from build123d import *

# Parameters (mm, degrees)
SKETCH2_W           = 5
SKETCH2_H           = 3
BOSS_EXTRUDE2_DEPTH = 10
BOSS_EXTRUDE3_DEPTH = 5


with BuildPart() as part:
    # Sketch2 → Boss-Extrude2 (new body)
    with BuildSketch(Plane(origin=(0, 0, 0), x_dir=(1, 0, 0), z_dir=(0, 1, 0))):
        Polygon((0, 40.223426607), (0, 50.279283258), (-20.111713303, 34.834509269), (-25.139641629, 43.543136586), (-34.834509269, 20.111713303), (-43.543136586, 25.139641629), (-40.223426607, 0), (-50.279283258, 0), (-34.834509269, -20.111713303), (-43.543136586, -25.139641629), (-20.111713303, -34.834509269), (-25.139641629, -43.543136586), (0, -40.223426607), (0, -50.279283258), (20.111713303, -34.834509269), (25.139641629, -43.543136586), (34.834509269, -20.111713303), (43.543136586, -25.139641629), (40.223426607, 0), (50.279283258, 0), (34.834509269, 20.111713303), (43.543136586, 25.139641629), (20.111713303, 34.834509269), (25.139641629, 43.543136586), align=None)
        Rectangle(SKETCH2_W, SKETCH2_H, mode=Mode.SUBTRACT)
    extrude(amount=BOSS_EXTRUDE2_DEPTH)

    # Sketch3 → Boss-Extrude3 (add)
    with BuildSketch(Plane(origin=(0, 10, 0), x_dir=(1, 0, 0), z_dir=(0, 1, 0))):
        Polygon((0, 35.761861209), (-3.15, 6.933446407), (3.15, 6.933446407), align=None)
    extrude(amount=BOSS_EXTRUDE3_DEPTH)


solid = part.part
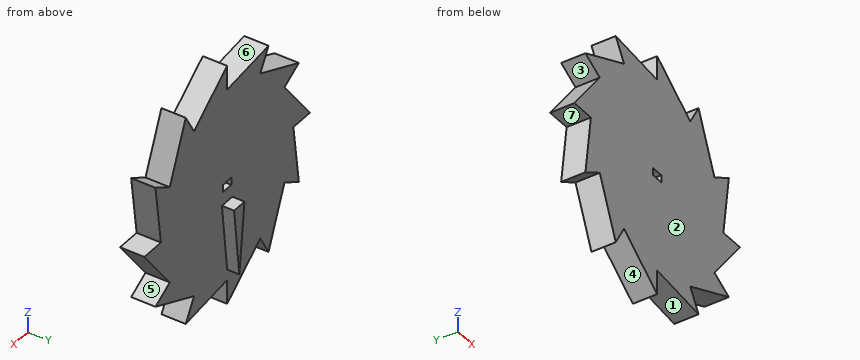
CAD build for the part. Positions are in the model's coordinates, mm. Face numbers are marked on the shaded views. A direction names the side the tool comes from. Give positions to 0.01 mm unless a question says otherwise; leave off trailing zeros. Write each loop counter-clockwise with the first axis right and the second up, starting at its lowest first coordinate (ties: lowest second). Pieces come first, ordered by that corner, then holes. Notation, with made-up numbers: (-30, -28.75) - (-12, -28.75) arc R36 ccw to (-12, 5.25) - close; hole circle Ø4 at (-11.75, 19.5). An arc over 180 degrees is marked (long way). Answer as CSV lines item,"result".
Q1. Band-saw the part on A-A (y = 7.5). Give the cut face in (x, z), and give its area (3 significant figures).
Result set:
outline,"(-50.28, 0) - (-40.22, 0) - (-43.54, -25.14) - (-34.83, -20.11) - (-25.14, -43.54) - (-20.11, -34.83) - (0, -50.28) - (0, -40.22) - (25.14, -43.54) - (20.11, -34.83) - (43.54, -25.14) - (34.83, -20.11) - (50.28, 0) - (40.22, 0) - (43.54, 25.14) - (34.83, 20.11) - (25.14, 43.54) - (20.11, 34.83) - (0, 50.28) - (0, 40.22) - (-25.14, 43.54) - (-20.11, 34.83) - (-43.54, 25.14) - (-34.83, 20.11) - close; hole (-2.5, -1.5) - (2.5, -1.5) - (2.5, 1.5) - (-2.5, 1.5) - close"
area,"6,050 mm²"
Q2. Drill centre lines: line 1 (Y direction, x = -21, z = 5); line 2 (Z direction, x = -35.5, y = 2.25); line 3 (Z direction, x = 35.5, y = 6.75). Where is each one in solid material? Low to high. Write a range as from..to.
Result set:
line 1,"0..10"
line 2,"-20.5..19.25, 20.5..28.47"
line 3,"-28.47..-20.5, -19.25..20.5"
Q3. Flat gauge pins, fed straight in: pin 1 Ø8 at (y, z) = (3.5, 42.5) entering from -X; pin 2 Ø5 at (y, z) = (5.5, -44.5) entering from +X; pin 3 Ø5.5 at (x, y) = (-0.5, 4.5) entering from -Z; pin 4 Ø6 at (x, y) = (31.5, 13.5) entering from -Z. Where does each tip first touch, or does it go through?
Result set:
pin 1,"x = -25.14"
pin 2,"x = 25.14"
pin 3,"z = -50.28"
pin 4,"through"
Q4. Pull direction Z, two halves, no side cores. Call the marked faces 1, 2 and 3: released by +Z, released by -Z, zero draft, split by the parting line, or undercut.
Result set:
face 1,"released by -Z"
face 2,"zero draft"
face 3,"undercut"
Q5. 3-axis set-ups, long thin cutter, end or side, ignore diameter. For the marked faces 4, 5, 6 and 7: which of +Z, -Z, +X, -X, +Y, -Y reach the whole face in a straight line?
Result set:
face 4,"-Z, +Y, -Y"
face 5,"+X, +Y, -Y"
face 6,"+Z, +Y, -Y"
face 7,"-X, +Y, -Y"
Q6. Band-saw the part on D-D (z = -11.5). Give the cut face in (x, y), and give its area (3 significant figures).
Result set:
outline,"(-41.74, 0) - (41.45, 0) - (41.45, 10) - (2.65, 10) - (2.65, 15) - (-2.65, 15) - (-2.65, 10) - (-41.74, 10) - close"
area,"858 mm²"
Q7. Band-saw the part on C-C (x = -23). Give the cut face in (y, z), and give its area (3 significant figures).
Result set:
outline,"(0, -39.84) - (10, -39.84) - (10, 33.64) - (0, 33.64) - close; (0, 39.84) - (10, 39.84) - (10, 43.26) - (0, 43.26) - close"
area,"769 mm²"
Q8. Band-saw the part on B-B (z = -37.5). Give the cut face in (x, y), and give its area (3 significant figures).
Result set:
outline,"(-27.64, 0) - (-21.65, 0) - (-21.65, 10) - (-27.64, 10) - close; (-16.64, 0) - (21.65, 0) - (21.65, 10) - (-16.64, 10) - close"
area,"443 mm²"
